For this review, take the finished solid that the model builds, in its own axes (mm). Coordinates: 2 decimals unless noted, no trailing zeros. Loops run counter-clockwise (first coordinate to the right, second up) from the corner with the lowest first, then second, coordinate; pieces in that order, holes last.
1. To check wall thickness, follow probe 1 along X at (y, z) = (270, -0.75); probe 2 along Y at (x, z) = (-0.5, -3.75); probe 3 along Z at (x, y) = (0.75, 577.5). State the ranges of each line that lie inside material, in increasing order.
2. Clearance check with flat-ended pins moving along their axes: P1, Ø3, axis at y = 507.5, z = 4.5, coming from the +X side; P2, Ø2, axis at x = -3.5, y = 601, coming from the +Z side; P3, Ø3, axis at y = 117, z = -5.5, coming from the +X side. State where each tip first meets the part, or that it passes through.
3. Take a section at A-A, the plane y = 384. State the section outline as (x, z) points, then the cut area to 3 significant figures.
4. Take a section at B-B, the plane y = 554. State the section outline as (x, z) points, then the cut area to 3 significant figures.
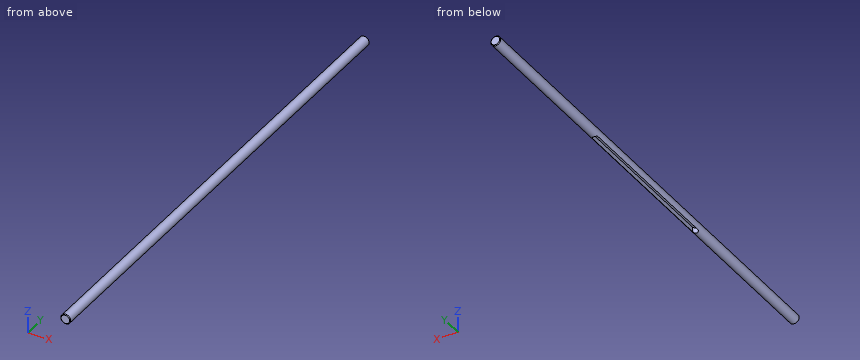
```python
from build123d import *

# Parameters (mm, degrees)
ESQUISSE1_R             = 7
BOSS_EXTRU_1_DEPTH      = 710
CHANFREIN1_SIZE         = 1
ENL_V_START             = 1
ENL_V_MAT_EXTRU_1_DEPTH = 10


with BuildPart() as part:
    # Esquisse1 → Boss.-Extru.1 (new body)
    with BuildSketch(Plane(origin=(0, 0, 0), x_dir=(1, 0, 0), z_dir=(0, 1, 0))):
        with Locations(Location((0, 0, 0), (0, 0, 270))):  # turned: the seam where the file's is
            Circle(ESQUISSE1_R)
    extrude(amount=BOSS_EXTRU_1_DEPTH)

    # Chanfrein1
    chanfrein1_edges = [part.edges().sort_by_distance(p)[0] for p in [
        (0, 0, -7),
        (0, 710, -7),
    ]]
    chamfer(chanfrein1_edges, length=CHANFREIN1_SIZE)

    # Esquisse2 → Enlèv. mat.-Extru.1 (cut)
    with BuildSketch(Plane.XY.offset(ENL_V_START)):
        with BuildLine():
            Line((-4, 473), (-4, 236))
            ThreePointArc((-4, 236), (0, 232), (4, 236))
            Line((4, 236), (4, 473))
            ThreePointArc((4, 473), (0, 477), (-4, 473))
        make_face()
    extrude(amount=-ENL_V_MAT_EXTRU_1_DEPTH, mode=Mode.SUBTRACT)


solid = part.part
```
Results list:
1. probe 1: x = -6.96 to -4, 4 to 6.96
1. probe 2: y = 0 to 232.03, 476.97 to 710
1. probe 3: z = -6.96 to 6.96
2. P1: stops at x = 6.32
2. P2: stops at z = 6.54
2. P3: stops at x = 5.74
3. outline: (-4, -5.74) - (-4, 1) - (4, 1) - (4, -5.74) arc R7 ccw (long way) to start
3. area: 93.2 mm2
4. outline: circle Ø14 at (0, 0)
4. area: 154 mm2
